Could you check a few things on this model? Use its own coordinates, in mm. Round coordinates to 2 decimals unless told otherwise and drop trailing zeros. Order: outer loops, then holes, each group sorted by start corner. A loop starts at its lowest first (then second) coordinate and runs counter-clockwise, first axis right, second up. Notation, with made-up numbers: (39.25, 44) -> (79.25, 44) arc R6 ccw to (79.25, 54) -> close; hole circle Ø3 at (17.5, 37). An arc over 180 degrees is marked (long way). One line per question, with ' | ' between items.
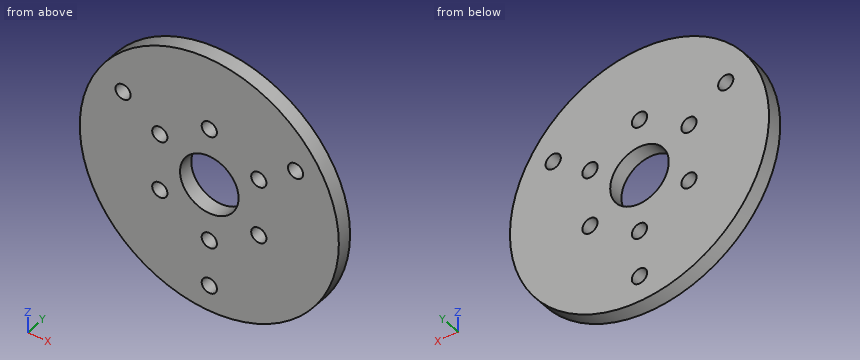
```python
from build123d import *

# Parameters (mm, degrees)
SKETCH1_R           = 53.975
SKETCH1_R_2         = 3.175
BOSS_EXTRUDE1_DEPTH = 6.35
SKETCH2_R           = 3.175
SKETCH2_R_2         = 12.2
CUT_EXTRUDE1_DEPTH  = 7.35


with BuildPart() as part:
    # Sketch1 → Boss-Extrude1 (new body)
    with BuildSketch(Plane(origin=(0, 0, 0), x_dir=(1, 0, 0), z_dir=(0, 1, 0))):
        Circle(SKETCH1_R)
        with Locations((0, 43.18)):
            Circle(SKETCH1_R_2, mode=Mode.SUBTRACT)
        with Locations((35.941, -22.86)):
            Circle(SKETCH1_R_2, mode=Mode.SUBTRACT)
        with Locations((-35.941, -22.86)):
            Circle(SKETCH1_R_2, mode=Mode.SUBTRACT)
    extrude(amount=BOSS_EXTRUDE1_DEPTH)

    # Sketch2 → Cut-Extrude1 (cut, through all)
    with BuildSketch(Plane(origin=(0, 6.35, 0), x_dir=(1, 0, 0), z_dir=(0, 1, 0))):
        with Locations((0, 23.8125)):
            Circle(SKETCH2_R)
        with Locations((20.622229928, 11.90625)):
            Circle(SKETCH2_R)
        with Locations((20.622229928, -11.90625)):
            Circle(SKETCH2_R)
        with Locations((0, -23.8125)):
            Circle(SKETCH2_R)
        with Locations((-20.622229928, -11.90625)):
            Circle(SKETCH2_R)
        with Locations((-20.622229928, 11.90625)):
            Circle(SKETCH2_R)
        Circle(SKETCH2_R_2)
    extrude(amount=-CUT_EXTRUDE1_DEPTH, mode=Mode.SUBTRACT)


solid = part.part
```
1. I want a section at A-A on z = 0. List the corners of the cut face in (x, y) for me (3 decimals).
From the geometry:
outline: (-53.975, 0) -> (-12.2, 0) -> (-12.2, 6.35) -> (-53.975, 6.35) -> close; (12.2, 0) -> (53.975, 0) -> (53.975, 6.35) -> (12.2, 6.35) -> close
2. I'm going to push flat-ended pins straight in: pin 1 (1.5 mm diameter, centred on x = 14.5, y = 1.5, fed in from -Z); pin 2 (1 mm diameter, centred on y = 1, z = 30, fed in from +X); pin 3 (2 mm diameter, centred on x = 42.5, y = 1.5, fed in from -Z); pin 4 (5.5 mm diameter, centred on x = 0, z = -23.81, fed in from -Y). Where does each tip first touch, or does it pass through?
From the geometry:
pin 1: stops at z = -52.19 | pin 2: stops at x = 45.2 | pin 3: stops at z = -34.51 | pin 4: passes through
3. I want a section at B-B on x = 0. Count the separate pieces of the cut face and the enclosed holes in it, and give its area (3 significant figures).
From the geometry:
separate pieces: 5 | enclosed holes: 0 | area: 410 mm²
4. I want a section at D-D on x = -19. List the corners of the cut face in (y, z) for me, and give its area (3 significant figures).
From the geometry:
outline: (0, -50.52) -> (6.35, -50.52) -> (6.35, -14.64) -> (0, -14.64) -> close; (0, -9.18) -> (6.35, -9.18) -> (6.35, 9.18) -> (0, 9.18) -> close; (0, 14.64) -> (6.35, 14.64) -> (6.35, 50.52) -> (0, 50.52) -> close | area: 572 mm²
5. I need wall thicknesses on probe 1 along Z at (x, y) = (0, 2.5) (1 decimal); probe 2 along X at (y, z) = (2.5, 22.86) (3 decimals); probe 3 along X at (y, z) = (4, 0.5). Which ranges of each line are inside material? Lowest first, please.
From the geometry:
probe 1: z = -54 to -46.4, -40 to -27, -20.6 to -12.2, 12.2 to 20.6, 27 to 54 | probe 2: x = -48.895 to -39.116, -32.766 to -3.029, 3.029 to 32.766, 39.116 to 48.895 | probe 3: x = -53.97 to -12.19, 12.19 to 53.97
